```python
from build123d import *

# Parameters (mm, degrees)
CUT_EXTRUDE1_REACH = 33.069
SKETCH3_R          = 2
FILLET1_R          = 2


with BuildPart() as part:
    # Sketch2 → Revolve1 (revolve)
    with BuildSketch(Plane(origin=(0, 0, 0), x_dir=(0, 0, -1), z_dir=(1, 0, 0)), mode=Mode.PRIVATE) as revolve1_sk:
        Polygon((0, 17), (0, 20.8), (-2, 20.8), (-10, 7.5), (-10, 3.55), (0, 3.55), (0, 5.3), (-7.6, 5.3), (-7.6, 7.5), (-2, 17), align=None)
    revolve(revolve1_sk.sketch.rotate(Axis((0, 0, 0), (0, 0, 1)), 90), axis=Axis((0, 0, 0), (0, 0, 1)))

    # Cut-Extrude1: up to this cone (the profile starts inside it)
    cut_extrude1_end = Plane(origin=(0, 0, 0), z_dir=(0, 0, -1)).offset(-14.511277195) * Cone(1.663e-06, 120.041275, 72.205277195, align=(Align.CENTER, Align.CENTER, Align.MIN), mode=Mode.PRIVATE)
    # Sketch3 → Cut-Extrude1 (cut, up to the surface)
    with BuildSketch(Plane.XY, mode=Mode.PRIVATE) as cut_extrude1_sk1:
        with Locations((0, 20.8)):
            Circle(SKETCH3_R)
    cut_extrude1_tool1 = extrude(cut_extrude1_sk1.sketch, amount=CUT_EXTRUDE1_REACH, mode=Mode.PRIVATE) & cut_extrude1_end
    add(cut_extrude1_tool1.solids().sort_by_distance((0, 20.8, 0))[0], mode=Mode.SUBTRACT)
    # Sketch3 → Cut-Extrude1 (cut, up to the surface)
    with BuildSketch(Plane.XY, mode=Mode.PRIVATE) as cut_extrude1_sk2:
        with Locations((20.8, 0)):
            Circle(SKETCH3_R)
    cut_extrude1_tool2 = extrude(cut_extrude1_sk2.sketch, amount=CUT_EXTRUDE1_REACH, mode=Mode.PRIVATE) & cut_extrude1_end
    add(cut_extrude1_tool2.solids().sort_by_distance((20.8, 0, 0))[0], mode=Mode.SUBTRACT)
    # Sketch3 → Cut-Extrude1 (cut, up to the surface)
    with BuildSketch(Plane.XY, mode=Mode.PRIVATE) as cut_extrude1_sk3:
        with Locations((0, -20.8)):
            Circle(SKETCH3_R)
    cut_extrude1_tool3 = extrude(cut_extrude1_sk3.sketch, amount=CUT_EXTRUDE1_REACH, mode=Mode.PRIVATE) & cut_extrude1_end
    add(cut_extrude1_tool3.solids().sort_by_distance((0, -20.8, 0))[0], mode=Mode.SUBTRACT)
    # Sketch3 → Cut-Extrude1 (cut, up to the surface)
    with BuildSketch(Plane.XY, mode=Mode.PRIVATE) as cut_extrude1_sk4:
        with Locations((-20.8, 0)):
            Circle(SKETCH3_R)
    cut_extrude1_tool4 = extrude(cut_extrude1_sk4.sketch, amount=CUT_EXTRUDE1_REACH, mode=Mode.PRIVATE) & cut_extrude1_end
    add(cut_extrude1_tool4.solids().sort_by_distance((-20.8, 0, 0))[0], mode=Mode.SUBTRACT)

    # Fillet1
    fillet1_edges = [part.edges().sort_by_distance(p)[0] for p in [
        (7.5, 0, 10),
    ]]
    fillet(fillet1_edges, radius=FILLET1_R)


solid = part.part
```
For this review, take the finished solid that the model builds, in its own axes (mm). A direction names the side the tool comes from. Round coordinates to 2 decimals unless told otherwise and drop trailing zeros. Write each loop counter-clockwise with the first axis right and the second up, starting at its lowest first coordinate (ties: lowest second). Pieces come first, ordered by that corner, then holes. Notation, with made-up numbers: (29.25, 5) - (76.25, 5) arc R21 cw to (76.25, 32) - close; hole circle Ø1 at (45.5, 12.25). An arc over 180 degrees is marked (long way). Answer as CSV lines item,"result". Start each with the question number.
(1) Add section D-D, the plane z = 5. State how many separate pieces and enclosed holes the cut face has, plus the area to 3 significant figures.
(2) Add section A-A, the plane z = 1.5. State the section outline as (x, y) points, plus the area to 3 significant figures.
(3) Machinability: for faces 5 (the flat face through (5, 3, 7.6)), 6 (the cylindrical face through (0, 18.8, 1.2)), which of the approach directions +Z, -Z, +X, -X, +Y, -Y give a long, thin tool a straight path to every point of the face, cutting with its end or side? Answer none if there is none.
(4) Add section B-B, the plane x = 0. State the section outline as (y, z) points.
(5) For line 1 (Y direction, x = 0, z = 0.9); line 2 (X direction, y = -2.5, z = 1.5); line 3 (X direction, y = 7.5, z = 0.75), list the stretches that pass through material, from the lowest coordinate up.
(6) Mouldability with a two-part tool opening along X and no side actions: class faces 1 (the cylindrical face through (14.849, 14.565, 1.014)), 2 (the cylindrical face through (4.21, 3.22, 3.85)), 3 (the cylindrical face through (-14.849, -14.565, 1.014)), 4 (the flat face through (-3, 3, 10)) as +X half, -X half, draft (parallel to the pull), parting line (faces both ways), or undercut.
(7) For pin 1 (2 mm diameter, centred on x = 3.5, y = -9.5, fed in from -Z); pin 2 (4 mm diameter, centred on x = 11.5, y = -5.5, fed in from +Z); pin 3 (1.5 mm diameter, centred on x = 7, y = -9.5, fed in from +Z), all flat-tipped, find the tip position at first contact; note any pin that passes through.
From the geometry:
1,separate pieces,"2"
1,enclosed holes,"2"
1,area,"388 mm²"
2,outline,"(-20.7, -2) arc R20.8 ccw to (-2, -20.7) arc R2 cw to (2, -20.7) arc R20.8 ccw to (20.7, -2) arc R2 cw to (20.7, 2) arc R20.8 ccw to (2, 20.7) arc R2 cw to (-2, 20.7) arc R20.8 ccw to (-20.7, 2) arc R2 cw to start; circle Ø10.6 at (0, 0); hole circle Ø34 at (0, 0); hole circle Ø7.1 at (0, 0)"
2,area,"475 mm²"
3,face 5,"-Z"
3,face 6,"+Z, -Z, +Y"
4,outline,"(-18.8, 0) - (-17, 0) - (-17, 2) - (-7.5, 7.6) - (-5.3, 7.6) - (-5.3, 0) - (-3.55, 0) - (-3.55, 10) - (-6.94, 10) arc R2 ccw to (-7.98, 9.71) - (-18.8, 3.2) - close; (3.55, 0) - (5.3, 0) - (5.3, 7.6) - (7.5, 7.6) - (17, 2) - (17, 0) - (18.8, 0) - (18.8, 3.2) - (7.98, 9.71) arc R2 ccw to (6.94, 10) - (3.55, 10) - close"
5,line 1,"y = -18.8 to -17, -5.3 to -3.55, 3.55 to 5.3, 17 to 18.8"
5,line 2,"x = -20.65 to -16.82, -4.67 to -2.52, 2.52 to 4.67, 16.82 to 20.65"
5,line 3,"x = -19.4 to -15.26, 15.26 to 19.4"
6,face 1,"+X half"
6,face 2,"undercut"
6,face 3,"-X half"
6,face 4,"draft"
7,pin 1,"stops at z = 5.46"
7,pin 2,"stops at z = 8.05"
7,pin 3,"stops at z = 7.86"
